from build123d import *

# Parameters (mm, degrees)
SKETCH1_W           = 58
SKETCH1_H           = 42
SKETCH1_W_2         = 42
SKETCH1_H_2         = 26
BOSS_EXTRUDE1_DEPTH = 30
SKETCH2_W           = 58
SKETCH2_H           = 42
BOSS_EXTRUDE2_DEPTH = 5
SKETCH4_R           = 1.75
CUT_EXTRUDE2_DEPTH  = 8
SKETCH5_R           = 1.75
CUT_EXTRUDE3_DEPTH  = 8
SKETCH6_R           = 2
CUT_EXTRUDE4_DEPTH  = 8
CUT_EXTRUDE5_START  = 42
SKETCH7_R           = 3
CUT_EXTRUDE5_DEPTH  = 3
SKETCH8_W           = 38.12950039
SKETCH8_H           = 31.187364713
BOSS_EXTRUDE3_DEPTH = 35
SKETCH9_R           = 5.2
CUT_EXTRUDE6_DEPTH  = 89.074186757
SKETCH10_R          = 1.65
CUT_EXTRUDE7_DEPTH  = 15
FILLET1_R           = 10
CUT_EXTRUDE8_DEPTH  = 89.074186757
BOSS_EXTRUDE4_DEPTH = 35
FILLET2_R           = 10
SKETCH13_R          = 1.6
CUT_EXTRUDE9_DEPTH  = 15
SKETCH14_R          = 6.6
CUT_EXTRUDE10_DEPTH = 5
SKETCH15_W          = 12
SKETCH15_H          = 8
CUT_EXTRUDE11_DEPTH = 99.51675752
FILLET3_R           = 5


with BuildPart() as part:
    # Sketch1 → Boss-Extrude1 (new body)
    with BuildSketch(Plane.XY):
        Rectangle(SKETCH1_W, SKETCH1_H)
        Rectangle(SKETCH1_W_2, SKETCH1_H_2, mode=Mode.SUBTRACT)
    extrude(amount=BOSS_EXTRUDE1_DEPTH)

    # Sketch2 → Boss-Extrude2 (add)
    with BuildSketch(Plane(origin=(0, 0, 0), x_dir=(-1, 0, 0), z_dir=(0, 0, -1))):
        Rectangle(SKETCH2_W, SKETCH2_H)
    extrude(amount=BOSS_EXTRUDE2_DEPTH)

    # Sketch4 → Cut-Extrude2 (cut)
    with BuildSketch(Plane.ZY.offset(29)):
        with Locations(Location((22.5, 10, 0), (0, 0, 270))):
            Circle(SKETCH4_R)
        with Locations(Location((22.5, -10, 0), (0, 0, 270))):
            Circle(SKETCH4_R)
    extrude(amount=-CUT_EXTRUDE2_DEPTH, mode=Mode.SUBTRACT)

    # Sketch5 → Cut-Extrude3 (cut)
    with BuildSketch(Plane.ZY.offset(29)):
        with Locations(Location((2.5, 10, 0), (0, 0, 270))):
            Circle(SKETCH5_R)
        with Locations(Location((2.5, -10, 0), (0, 0, 270))):
            Circle(SKETCH5_R)
    extrude(amount=-CUT_EXTRUDE3_DEPTH, mode=Mode.SUBTRACT)

    # Sketch6 → Cut-Extrude4 (cut)
    with BuildSketch(Plane.ZY.offset(29)):
        with Locations(Location((22.5, 10, 0), (0, 0, 270))):
            Circle(SKETCH6_R)
        with Locations(Location((2.5, 10, 0), (0, 0, 270))):
            Circle(SKETCH6_R)
        with Locations(Location((2.5, -10, 0), (0, 0, 270))):
            Circle(SKETCH6_R)
        with Locations(Location((22.5, -10, 0), (0, 0, 270))):
            Circle(SKETCH6_R)
    extrude(amount=-CUT_EXTRUDE4_DEPTH, mode=Mode.SUBTRACT)

    # Sketch7 → Cut-Extrude5 (cut)
    with BuildSketch(Plane.ZY.offset(-21).offset(CUT_EXTRUDE5_START)):
        with Locations(Location((22.5, 10, 0), (0, 0, 90))):
            Circle(SKETCH7_R)
        with Locations(Location((22.5, -10, 0), (0, 0, 180))):
            Circle(SKETCH7_R)
        with Locations(Location((2.5, 10, 0), (0, 0, 90))):
            Circle(SKETCH7_R)
        with Locations(Location((2.5, -10, 0), (0, 0, 146.442690238))):
            Circle(SKETCH7_R)
    extrude(amount=CUT_EXTRUDE5_DEPTH, mode=Mode.SUBTRACT)

    # Sketch8 → Boss-Extrude3 (add)
    with BuildSketch(Plane.XY.offset(30)):
        with Locations((-48.064750195, 29.414011989)):
            Rectangle(SKETCH8_W, SKETCH8_H)
    extrude(amount=-BOSS_EXTRUDE3_DEPTH)

    # Sketch9 → Cut-Extrude6 (cut, through all)
    with BuildSketch(Plane.XY.offset(30)):
        with Locations((-52.000004001, 30.827632123)):
            Circle(SKETCH9_R)
    extrude(amount=-CUT_EXTRUDE6_DEPTH, mode=Mode.SUBTRACT)

    # Sketch10 → Cut-Extrude7 (cut)
    with BuildSketch(Plane.XY.offset(30)):
        with Locations((-45.750541353, 35.822050669)):
            Circle(SKETCH10_R)
        with Locations((-47.005585454, 24.578169475)):
            Circle(SKETCH10_R)
        with Locations((-56.994422547, 37.07709477)):
            Circle(SKETCH10_R)
        with Locations((-58.249466648, 25.833213576)):
            Circle(SKETCH10_R)
    extrude(amount=-CUT_EXTRUDE7_DEPTH, mode=Mode.SUBTRACT)

    # Fillet1
    fillet1_edges = [part.edges().sort_by_distance(p)[0] for p in [
        (-67.12950039, 45.007694345, 12.5),
        (-67.12950039, 13.820329632, 12.5),
        (-29, 45.007694345, 12.5),
        (-29, 21, 12.5),
        (29, 21, 12.5),
        (29, -21, 12.5),
    ]]
    fillet(fillet1_edges, radius=FILLET1_R)

    # Sketch11 → Cut-Extrude8 (cut, through all)
    with BuildSketch(Plane.XY.offset(30)):
        with BuildLine():
            Line((-57.12950039, 13.820329632), (-29, 13.820329632))
            add(Edge.make_bspline(
                [(-52.000004001, 19.827632123), (-39.662764049, 19.484687558), (-29, 13.820329632)],
                knots=[0, 0, 0, 1, 1, 1], degree=2))
            ThreePointArc((-52.000004001, 19.827632123), (-62.690470456, 33.418756776), (-46.963580148, 40.606918128))
            add(Edge.make_bspline(
                [(-29, 31), (-36.987178252, 37.635549332), (-46.963580148, 40.606918128)],
                knots=[0, 0, 0, 1, 1, 1], degree=2))
            Line((-29, 31), (-29, 35.007694345))
            ThreePointArc((-29, 35.007694345), (-31.928932188, 42.078762157), (-39, 45.007694345))
            Line((-39, 45.007694345), (-57.12950039, 45.007694345))
            ThreePointArc((-57.12950039, 45.007694345), (-64.200568202, 42.078762157), (-67.12950039, 35.007694345))
            Line((-67.12950039, 35.007694345), (-67.12950039, 23.820329632))
            ThreePointArc((-67.12950039, 23.820329632), (-64.200568202, 16.74926182), (-57.12950039, 13.820329632))
        make_face()
    extrude(amount=-CUT_EXTRUDE8_DEPTH, mode=Mode.SUBTRACT)

    # Sketch12 → Boss-Extrude4 (add)
    with BuildSketch(Plane.XY.offset(30)):
        with BuildLine():
            Line((-29, 31), (-19, 21))
            ThreePointArc((-19, 21), (-26.071067812, 23.928932188), (-29, 31))
        make_face()
    extrude(amount=-BOSS_EXTRUDE4_DEPTH)

    # Fillet2
    fillet2_edges = [part.edges().sort_by_distance(p)[0] for p in [
        (-19, 21, 12.5),
    ]]
    fillet(fillet2_edges, radius=FILLET2_R)

    # Sketch13 → Cut-Extrude9 (cut)
    with BuildSketch(Plane.XY.offset(30)):
        with Locations((24.65, 4.935)):
            Circle(SKETCH13_R)
        with Locations((24.65, -4.935)):
            Circle(SKETCH13_R)
        with Locations((-24.65, 4.935)):
            Circle(SKETCH13_R)
        with Locations((-24.65, -4.935)):
            Circle(SKETCH13_R)
    extrude(amount=-CUT_EXTRUDE9_DEPTH, mode=Mode.SUBTRACT)

    # Sketch14 → Cut-Extrude10 (cut)
    with BuildSketch(Plane(origin=(0, 0, -5), x_dir=(-1, 0, 0), z_dir=(0, 0, -1))):
        with Locations((-10.250000003, -1e-09)):
            Circle(SKETCH14_R)
    extrude(amount=-CUT_EXTRUDE10_DEPTH, mode=Mode.SUBTRACT)

    # Sketch15 → Cut-Extrude11 (cut, through all)
    with BuildSketch(Plane.ZY.offset(-21)):
        with Locations((6, 0)):
            Rectangle(SKETCH15_W, SKETCH15_H)
    extrude(amount=-CUT_EXTRUDE11_DEPTH, mode=Mode.SUBTRACT)

    # Fillet3
    fillet3_edges = [part.edges().sort_by_distance(p)[0] for p in [
        (-29, -21, 12.5),
    ]]
    fillet(fillet3_edges, radius=FILLET3_R)


solid = part.part
CAD build for the part. Positions are in the model's coordinates, mm. A direction names the side the tool comes from. Give positions to 0.01 mm unless a question says otherwise; leave off trailing zeros. Write each loop counter-clockwise with the first axis right and the second up, starting at its lowest first coordinate (ties: lowest second). Pieces come first, ordered by that corner, then holes. Notation, with made-up numbers: M 35,10 L 87,10 A28 cw 87,37 Z; hole C 81,-4 d5. An arc over 180 degrees is marked long. Put each result on its own line as item: value. Start each with the question number.
(1) Flat gauge pins, fed straight in: pin 1 Ø1.9 at (x, y) = (-24.65, -4.935) entering from +Z; pin 2 Ø6 at (x, z) = (-7.5, 26) entering from +Y; pin 3 Ø1 at (x, z) = (-33, 8.5) entering from -Y; pin 4 Ø10.5 at (x, y) = (10.25, 0) entering from +Z. Where does each tip first touch, or does it go through?
(2) Probe L1, parallel to X at y = 9, z = 14; L2, parallel to Y at x = -2, z = 10.5; L3, parallel to Y at x = 11, z = -2. List the from-to ranges inside material, lowest first.
(3) Which spindle directions (+Z, -Z, +X, -X, +Y, -Y) get a long thin tool onto all of the face, cutting with end or side? Do faces 5 (the face through (0, -13, 15)), 6 (the face through (2, 21, 13)), 7 (the face through (-29, -1, 13)), 8 (the face through (3.955, 1.982, -2.535)), 9 (the face through (-24, -8, 1)). Say none if no direction does.
(4) Band-saw the part on D-D, the plane x = -11. Write the cut outline in (y, z).
(5) Mould opens along X. For faces 1 (the face through (-22.48, 12.86, 1.6)), 2 (the face through (-26.5, 11.6, 1.3)), 3 (the face through (25.99, 18.15, 12.74)), 4 (the face through (-25.829, -3.854, 22.605)) say: +X half, -X half, draft (parallel to the pull), parting line (faces both ways), or undercut.
(6) Band-saw the part on A-A, the plane y = -10. Write the cut outline in (x, z).
(7) Band-saw the part on C-C, the plane y = 0. Write the cut outline in (x, z).
(8) Band-saw the part on B-B, the plane x = 10.25. Write the cut outline in (y, z), and give its area (3 significant figures).
Response values:
1. pin 1: stops at z = 15
1. pin 2: stops at y = 21
1. pin 3: stops at y = 15.52
1. pin 4: passes through
2. L1: x = -29 to -21, 21 to 29
2. L2: y = -21 to -13, 13 to 21
2. L3: y = -21 to -6.56, 6.56 to 21
3. face 5: +Z
3. face 6: +Z, -Z, +X, +Y
3. face 7: +Z, -Z, -X, -Y
3. face 8: +Z, -Z
3. face 9: none
4. outline: M -21,-5 L 21,-5 L 21,30 L 13,30 L 13,0 L -13,0 L -13,30 L -21,30 Z
5. face 1: undercut
5. face 2: draft
5. face 3: +X half
5. face 4: undercut
6. outline: M -29,-5 L 29,-5 L 29,30 L 21,30 L 21,0 L -21,0 L -21,-0.5 L -24,-0.5 L -24,0.5 L -29,0.5 Z; M -29,4.5 L -24,4.5 L -24,5.5 L -21,5.5 L -21,19.5 L -24,19.5 L -24,20.5 L -29,20.5 Z; M -29,24.5 L -24,24.5 L -24,25.5 L -21,25.5 L -21,30 L -29,30 Z
7. outline: M -29,-5 L 3.65,-5 L 3.65,0 L -21,0 L -21,30 L -29,30 Z; M 16.85,-5 L 29,-5 L 29,0 L 16.85,0 Z; M 21,12 L 29,12 L 29,30 L 21,30 Z
8. outline: M -21,-5 L -6.6,-5 L -6.6,0 L -13,0 L -13,30 L -21,30 Z; M 6.6,-5 L 21,-5 L 21,30 L 13,30 L 13,0 L 6.6,0 Z
8. area: 624 mm2
